Geometry: final body of the model. Coordinates: model frame, mm. Coordinates: 2 decimals unless noted, no trailing zeros. Loops run counter-clockwise (first coordinate to the right, second up) from the corner with the lowest first, then second, coordinate; pieces in that order, holes last. Notation, with made-up numbers: (50, -38.75) - (61, -38.75) arc R11 cw to (61, -34.75) - close; hole circle Ø2 at (0, 72.25). An arc over 180 degrees is marked (long way). Return JSON: item names as keys, results as strings.
from build123d import *

# Parameters (mm, degrees)
WYTNIJ_WYCI_GNI_CIE1_DEPTH      = 12.643131022
WYTNIJ_WYCI_GNI_CIE1_DEPTH_BACK = 12.643131022
SZKIC2_R                        = 0.8


with BuildPart() as part:
    # Szkic1 → Obrót1 (revolve)
    with BuildSketch(Plane(origin=(0, 0, 0), x_dir=(1, 0, 0), z_dir=(0, 1, 0))):
        Polygon((0, -9.75), (4, -9.75), (4.5, -9.25), (4.5, -8.25), (3, -8.25), (3, 8.25), (2.133974596, 9.75), (0, 9.75), align=None)
    revolve(axis=Axis((0, 0, 9.75), (0, 0, -1)))

    # Szkic2 → Wytnij-wyciągnięcie1 (cut, two sides: drawn at the far end of the back side and taken through both)
    with BuildSketch(Plane(origin=(0, 0, 0), x_dir=(1, 0, 0), z_dir=(0, 1, 0)).offset(-WYTNIJ_WYCI_GNI_CIE1_DEPTH_BACK)):
        with Locations(Location((0, 7.05, 0), (0, 0, 270))):
            Circle(SZKIC2_R)
    extrude(amount=WYTNIJ_WYCI_GNI_CIE1_DEPTH + WYTNIJ_WYCI_GNI_CIE1_DEPTH_BACK, mode=Mode.SUBTRACT)


solid = part.part
Item 1: Mould query, pull axis Z, two halves, no side actions, for faces 1 (the face through (0, 0, -9.75)), 2 (the face through (-0.306, -0.042, -6.311)), 3 (the face through (0, 0, 9.75)), 4 (the face through (-0.59, -4.46, 8.74)). Classes: +Z half, -Z half, draft (parallel to the pull), parting line (faces both ways), or undercut.
Worked out:
{"face 1": "-Z half", "face 2": "undercut", "face 3": "+Z half", "face 4": "draft"}
Item 2: Section query A-A, the plane x = 0. Return loops of the section in (y, z), and give its area (3 significant figures).
Worked out:
{"outline": "(-4.5, 8.25) - (-3, 8.25) - (-3, -6.25) - (3, -6.25) - (3, 8.25) - (4.5, 8.25) - (4.5, 9.25) - (4, 9.75) - (-4, 9.75) - (-4.5, 9.25) - close; (-3, -8.25) - (-2.13, -9.75) - (2.13, -9.75) - (3, -8.25) - (3, -7.85) - (-3, -7.85) - close", "area": "110 mm^2"}
Item 3: Section query C-C, the plane z = 4. Return loops of the section in (x, y), and give its area (3 significant figures).
Worked out:
{"outline": "circle Ø6 at (0, 0)", "area": "28.3 mm^2"}
Item 4: First-contact query: pin 1 Ø1.5 at (y, z) = (2.5, -3) entering from -X; pin 2 Ø1.4 at (x, z) = (0, -7.05) entering from +Y; pin 3 Ø1.5 at (y, z) = (2, 3) entering from +X; pin 4 Ø1.5 at (y, z) = (-1, 4.5) entering from -X. Flat tips, straight axial feed; report the tip coordinate or a pass-through.
Worked out:
{"pin 1": "x = -2.44", "pin 2": "through", "pin 3": "x = 2.73", "pin 4": "x = -2.99"}
Item 5: Ray query, probe 1 along X at (y, z) = (0, -7.05); probe 2 along Z at (x, y) = (0, 0.25); probe 3 along X at (y, z) = (-0.75, -7.05). Return the intervals inside material, ascending. Write a range as from..to.
Worked out:
{"probe 1": "-3..-0.8, 0.8..3", "probe 2": "-9.75..-7.85, -6.25..9.75", "probe 3": "-2.9..-0.8, 0.8..2.9"}
Item 6: Section query B-B, the plane y = 0. Return loops of the section in (x, z).
Worked out:
{"outline": "(-4.5, 8.25) - (-3, 8.25) - (-3, -8.25) - (-2.13, -9.75) - (2.13, -9.75) - (3, -8.25) - (3, 8.25) - (4.5, 8.25) - (4.5, 9.25) - (4, 9.75) - (-4, 9.75) - (-4.5, 9.25) - close; hole circle Ø1.6 at (0, -7.05)"}
Item 7: Section query D-D, the plane z = -7.05. Return loops of the section in (x, y), and give its area (3 significant figures).
Worked out:
{"outline": "(-0.8, -2.89) - (-0.8, 2.89) arc R3 ccw to start; (0.8, -2.89) arc R3 ccw to (0.8, 2.89) - close", "area": "18.8 mm^2"}
